Source: CAD feature listing. Evaluate the final solid. Frame: model axes, mm. A direction names the side the tool comes from. Round coordinates to 2 decimals unless told otherwise and drop trailing zeros. Write each loop counter-clockwise with the first axis right and the second up, starting at its lowest first coordinate (ties: lowest second). Pieces come first, ordered by that corner, then holes. Notation, with made-up numbers: M -14,17.5 L -5,17.5 A16 cw -5,34.5 Z; hole C 32,-20 d10. An arc over 180 degrees is marked long. Answer in a Markdown table with one row per item. Add a question column.
Item 1: Cut plane C-C on x = 20. Return loops of the section in (y, z) (1 decimal), and give its area (3 significant figures).
Item 2: Cut plane D-D on y = 5.25. Give the number of separate pieces and of enclosed holes in the cut face, and give its area (3 significant figures).
Item 3: Cut plane A-A on z = 7.5. Return loops of the section in (x, y) (1 decimal).
Item 4: Mould query, pull axis Z, two halves, no side actions, for faces 1 (the face through (-28.575, 5, 0)), 2 (the face through (0, 5, 28.575)), 3 (the face through (-17, 3.175, 19)). Classes: released by +Z, released by -Z, zero draft, split by the parting line, or undercut.
Item 5: Set-up query: faces 4 (the face through (26.033, 11.917, 26.082)), 5 (the face through (-26.988, 12, 0)), 6 (the face through (-26.082, 11.917, 26.033)), 7 (the face through (24.315, 8.004, -10.404)). Return all of +Z, -Z, +X, -X, +Y, -Y with unobstructed straight access to the full face (end or side cutting, diameter ignored); none if empty.
Item 6: Contact query for flat-ended pins moving along their axis: pin 1 (2.5 mm diameter, centred on x = -16.5, z = -2, fed in from +Y); pin 2 (1.7 mm diameter, centred on x = -6.5, y = 12.5, fed in from -Z); pin 3 (0.5 mm diameter, centred on x = -1, y = 12, fed in from +Z). Output: stop coordinate, or through.
Item 7: Cut plane B-B on x = 0. Return loops of the section in (y, z) (1 decimal).
Item 8: Material intervals for probe 1 along Z at (x, y) = (-12.5, 7) (3 decimals); probe 2 along Z at (x, y) = (18, 8.5) (3 decimals); probe 3 along X at (y, z) = (9.5, 23) (3 decimals), sorted ascending.
from build123d import *

# Parameters (mm, degrees)
SKETCH1_W          = 57.15
SKETCH1_H          = 57.15
SKETCH1_R          = 14.2875
STOCK_DEPTH        = 12.7
SKETCH6_R          = 2.54
MOUNT_HOLES_DEPTH  = 43.359783404
SKETCH2_W          = 57.15
SKETCH2_H          = 57.15
LIP_DEPTH          = 1.5875
SKETCH4_R          = 10.31875
SKETCH4_R_2        = 3.175
BEARING_CUTS_DEPTH = 9.525
SKETCH5_R          = 22.225
INNER_RACE_DEPTH   = 0.79375
OUTER_START        = -0.79375
SKETCH8_R          = 22.225
OUTER_RACE_DEPTH   = 0.79375
FILLET1_R          = 1.5875


with BuildPart() as part:
    # Sketch1 → Stock (new body)
    with BuildSketch(Plane(origin=(0, 0, 0), x_dir=(1, 0, 0), z_dir=(0, 1, 0))):
        Rectangle(SKETCH1_W, SKETCH1_H)
        with Locations(Location((0, 0, 0), (0, 0, 270))):
            Circle(SKETCH1_R, mode=Mode.SUBTRACT)
    extrude(amount=STOCK_DEPTH)

    # Sketch6 → Mount Holes (cut, through all)
    with BuildSketch(Plane.XZ):
        with Locations(Location((-23.622, 23.622, 0), (0, 0, 270))):
            Circle(SKETCH6_R)
        with Locations(Location((23.622, 23.622, 0), (0, 0, 270))):
            Circle(SKETCH6_R)
        with Locations(Location((23.622, -23.622, 0), (0, 0, 270))):
            Circle(SKETCH6_R)
        with Locations(Location((-23.622, -23.622, 0), (0, 0, 270))):
            Circle(SKETCH6_R)
    extrude(amount=-MOUNT_HOLES_DEPTH, mode=Mode.SUBTRACT)

    # Sketch2 → Lip (cut)
    with BuildSketch(Plane(origin=(0, 12.7, 0), x_dir=(1, 0, 0), z_dir=(0, 1, 0))):
        Rectangle(SKETCH2_W, SKETCH2_H)
        with BuildLine():
            Line((-23.8125, -26.9875), (23.8125, -26.9875))
            ThreePointArc((23.8125, -26.9875), (26.05756403, -26.05756403), (26.9875, -23.8125))
            Line((26.9875, -23.8125), (26.9875, 23.8125))
            ThreePointArc((26.9875, 23.8125), (26.05756403, 26.05756403), (23.8125, 26.9875))
            Line((23.8125, 26.9875), (-23.8125, 26.9875))
            ThreePointArc((-23.8125, 26.9875), (-26.05756403, 26.05756403), (-26.9875, 23.8125))
            Line((-26.9875, 23.8125), (-26.9875, -23.8125))
            ThreePointArc((-26.9875, -23.8125), (-26.05756403, -26.05756403), (-23.8125, -26.9875))
        make_face(mode=Mode.SUBTRACT)
    extrude(amount=-LIP_DEPTH, mode=Mode.SUBTRACT)

    # Sketch4 → Bearing Cuts (cut)
    # profile 1 of 4: a face of its own
    with BuildSketch(Plane(origin=(0, 12.7, 0), x_dir=(1, 0, 0), z_dir=(0, 1, 0))):
        with Locations((15.154182204, 15.154182204)):
            Circle(SKETCH4_R)
        with Locations(Location((15.154182204, 15.154182204, 0), (0, 0, 270))):
            Circle(SKETCH4_R_2, mode=Mode.SUBTRACT)
    # profile 2 of 4: a face of its own
    with BuildSketch(Plane(origin=(0, 12.7, 0), x_dir=(1, 0, 0), z_dir=(0, 1, 0))):
        with Locations((15.154182204, -15.154182204)):
            Circle(SKETCH4_R)
        with Locations(Location((15.154182204, -15.154182204, 0), (0, 0, 270))):
            Circle(SKETCH4_R_2, mode=Mode.SUBTRACT)
    # profile 3 of 4: a face of its own
    with BuildSketch(Plane(origin=(0, 12.7, 0), x_dir=(1, 0, 0), z_dir=(0, 1, 0))):
        with Locations((-15.154182204, -15.154182204)):
            Circle(SKETCH4_R)
        with Locations(Location((-15.154182204, -15.154182204, 0), (0, 0, 270))):
            Circle(SKETCH4_R_2, mode=Mode.SUBTRACT)
    # profile 4 of 4: a face of its own
    with BuildSketch(Plane(origin=(0, 12.7, 0), x_dir=(1, 0, 0), z_dir=(0, 1, 0))):
        with Locations((-15.154182204, 15.154182204)):
            Circle(SKETCH4_R)
        with Locations(Location((-15.154182204, 15.154182204, 0), (0, 0, 270))):
            Circle(SKETCH4_R_2, mode=Mode.SUBTRACT)
    extrude(amount=-BEARING_CUTS_DEPTH, mode=Mode.SUBTRACT)

    # Sketch5 → Inner Race (cut)
    with BuildSketch(Plane(origin=(0, 12.7, 0), x_dir=(1, 0, 0), z_dir=(0, 1, 0))):
        Circle(SKETCH5_R)
    extrude(amount=-INNER_RACE_DEPTH, mode=Mode.SUBTRACT)

    # Sketch8 → Outer Race (cut)
    with BuildSketch(Plane.XZ.offset(OUTER_START)):
        with Locations(Location((0, 0, 0), (0, 0, 270))):
            Circle(SKETCH8_R)
    extrude(amount=OUTER_RACE_DEPTH, mode=Mode.SUBTRACT)

    # Fillet1
    fillet1_edges = [part.edges().sort_by_distance(p)[0] for p in [
        (-13.388674142, 7.540625, 4.987590699),
        (-4.987590699, 7.540625, -13.388674142),
        (-13.388674142, 7.540625, -4.987590699),
        (-4.987590699, 7.540625, 13.388674142),
        (13.388674142, 7.540625, 4.987590699),
        (4.987590699, 7.540625, -13.388674142),
        (13.388674142, 7.540625, -4.987590699),
        (4.987590699, 7.540625, 13.388674142),
    ]]
    fillet(fillet1_edges, radius=FILLET1_R)


solid = part.part
Results below:
| question | item | result |
|---|---|---|
| 1 | outline | M 0,-28.6 L 11.1,-28.6 L 11.1,-27 L 12.7,-27 L 12.7,-24.3 L 3.2,-24.3 L 3.2,-6 L 11.9,-6 L 11.9,6 L 3.2,6 L 3.2,24.3 L 12.7,24.3 L 12.7,27 L 11.1,27 L 11.1,28.6 L 0,28.6 L 0,9.7 L 0.8,9.7 L 0.8,-9.7 L 0,-9.7 Z |
| 1 | area | 349 mm2 |
| 2 | separate pieces | 5 |
| 2 | enclosed holes | 1 |
| 2 | area | 1,430 mm2 |
| 3 | outline | M -28.6,0 L -20.9,0 L -20.9,0.8 L -12.2,0.8 L -12.2,3.2 L -22.1,3.2 L -22.1,12.7 L -27,12.7 L -27,11.1 L -28.6,11.1 Z; M 12.2,0.8 L 20.9,0.8 L 20.9,0 L 28.6,0 L 28.6,11.1 L 27,11.1 L 27,12.7 L 22.1,12.7 L 22.1,3.2 L 12.2,3.2 Z |
| 4 | face 1 | zero draft |
| 4 | face 2 | released by +Z |
| 4 | face 3 | undercut |
| 5 | face 4 | +Z, +X, +Y |
| 5 | face 5 | +Z, -Z, -X, +Y |
| 5 | face 6 | +Z, -X, +Y |
| 5 | face 7 | +Y |
| 6 | pin 1 | y = 11.91 |
| 6 | pin 2 | z = -26.99 |
| 6 | pin 3 | z = 26.99 |
| 7 | outline | M 0,-28.6 L 11.1,-28.6 L 11.1,-27 L 12.7,-27 L 12.7,-22.2 L 11.9,-22.2 L 11.9,-14.3 L 0.8,-14.3 L 0.8,-22.2 L 0,-22.2 Z; M 0,22.2 L 0.8,22.2 L 0.8,14.3 L 11.9,14.3 L 11.9,22.2 L 12.7,22.2 L 12.7,27 L 11.1,27 L 11.1,28.6 L 0,28.6 Z |
| 8 | probe 1 | -28.575 to -25.126, -16.897 to -13.412, 13.412 to 16.897, 25.126 to 28.575 |
| 8 | probe 2 | -28.575 to -25.073, -16.562 to -13.746, -5.236 to 5.236, 13.746 to 16.562, 25.073 to 28.575 |
| 8 | probe 3 | -28.575 to -26.085, -8.452 to 8.452, 26.085 to 28.575 |
